CAD build for the part. Positions are in the model's coordinates, mm. Face numbers are marked on the shaded views. A direction names the side the tool comes from. Give positions to 0.01 mm unless a question says otherwise; leave off trailing zeros. Write each loop counter-clockwise with the first axis right and the second up, starting at its lowest first coordinate (ties: lowest second). Pieces come first, ordered by that corner, then holes. Notation, with made-up numbers: (43, 1) - (83, 1) arc R16 ccw to (83, 8) - close; hole circle Ø8 at (46, 48). An arc over 180 degrees is marked (long way). Answer as a JSON object with one key per item and string values.
from build123d import *

# Parameters (mm, degrees)
SKETCH1_W               = 56.4
SKETCH1_H               = 56.4
SKETCH1_R               = 2.5
SKETCH1_R_2             = 20
SKETCH1_W_2             = 42.3
SKETCH1_H_2             = 42.45
SKETCH1_R_3             = 1.25
SKETCH1_R_4             = 12.5
BOSS_EXTRUDE1_DEPTH     = 3
BOSS_EXTRUDE2_DEPTH     = 3
BOSS_EXTRUDE3_DEPTH     = 3
BOSS_EXTRUDE4_DEPTH     = 3
BOSS_EXTRUDE5_DEPTH     = 7.05
SKETCH6_W               = 62.4
SKETCH6_H               = 25
BOSS_EXTRUDE6_DEPTH     = 3
SKETCH7_W               = 55.35
SKETCH7_H               = 25
BOSS_EXTRUDE7_DEPTH     = 3
SKETCH8_W               = 26.348542459
SKETCH8_H               = 5
SKETCH8_W_2             = 28.376425856
SKETCH8_W_3             = 30.843971631
SKETCH8_W_4             = 29.425531915
BOSS_EXTRUDE8_DEPTH     = 60
SKETCH9_R               = 69.252729773
SKETCH9_R_2             = 19.252729773
CUT_EXTRUDE1_DEPTH      = 5
CUT_EXTRUDE2_START      = -51
SKETCH9_2_R             = 69.252729773
SKETCH9_2_R_2           = 19.252729773
CUT_EXTRUDE2_DEPTH      = 5
CUT_EXTRUDE3_DEPTH      = 136.205325339
CUT_EXTRUDE3_DEPTH_BACK = 136.205325339
SKETCH10_R              = 62.5
BOSS_EXTRUDE9_DEPTH     = 31
CUT_EXTRUDE4_DEPTH      = 129.360741662
CUT_EXTRUDE4_DEPTH_BACK = 129.360741662
SKETCH12_R              = 3


with BuildPart() as part:
    # Sketch1 → Boss-Extrude1 (new body)
    # profile 1 of 2: a face of its own
    with BuildSketch(Plane.XY):
        Rectangle(SKETCH1_W, SKETCH1_H)
        with Locations((-23.55, -23.55)):
            Circle(SKETCH1_R, mode=Mode.SUBTRACT)
        with Locations((-23.55, 23.55)):
            Circle(SKETCH1_R, mode=Mode.SUBTRACT)
        with Locations((23.55, 23.55)):
            Circle(SKETCH1_R, mode=Mode.SUBTRACT)
        with Locations((23.55, -23.55)):
            Circle(SKETCH1_R, mode=Mode.SUBTRACT)
        Circle(SKETCH1_R_2, mode=Mode.SUBTRACT)
    # profile 2 of 2: a face of its own
    with BuildSketch(Plane.XY):
        with Locations((0, 49.425)):
            Rectangle(SKETCH1_W_2, SKETCH1_H_2)
        with Locations((-15.49, 34)):
            Circle(SKETCH1_R_3, mode=Mode.SUBTRACT)
        with Locations((-15.49, 64.99)):
            Circle(SKETCH1_R_3, mode=Mode.SUBTRACT)
        with Locations((15.5, 64.99)):
            Circle(SKETCH1_R_3, mode=Mode.SUBTRACT)
        with Locations((15.5, 34)):
            Circle(SKETCH1_R_3, mode=Mode.SUBTRACT)
        with Locations((0, 49.5)):
            Circle(SKETCH1_R_4, mode=Mode.SUBTRACT)
    extrude(amount=BOSS_EXTRUDE1_DEPTH)

    # Sketch2 → Boss-Extrude2 (add)
    with BuildSketch(Plane.ZY.offset(28.2)):
        Polygon((-22, -28.2), (-30, 28.2), (0, 28.2), (3, 28.2), (3, -28.2), align=None)
    boss_extrude2 = extrude(amount=BOSS_EXTRUDE2_DEPTH)

    # Mirror1: Boss-Extrude2 across plane
    add(boss_extrude2.mirror(Plane(origin=(0, 0, 0), x_dir=(0, 0, 1), z_dir=(1, 0, 0))))

    # Sketch3 → Boss-Extrude3 (add)
    with BuildSketch(Plane(origin=(0, 28.2, 0), x_dir=(1, 0, 0), z_dir=(0, 1, 0))):
        Polygon((-21.1, 30), (-31.2, 30), (-31.2, -3), (31.2, -3), (31.2, 30), (21.1, 30), (21.1, 0), (-21.1, 0), align=None)
    extrude(amount=BOSS_EXTRUDE3_DEPTH)

    # Sketch4 → Boss-Extrude4 (add)
    with BuildSketch(Plane(origin=(21.15, 0, 0), x_dir=(0, 0, -1), z_dir=(1, 0, 0))):
        Polygon((30, 31.2), (22, 70.65), (-3, 70.65), (-3, 31.2), align=None)
    boss_extrude4 = extrude(amount=BOSS_EXTRUDE4_DEPTH)

    # Mirror2: Boss-Extrude4 across plane
    add(boss_extrude4.mirror(Plane(origin=(0, 0, 0), x_dir=(0, 0, 1), z_dir=(1, 0, 0))))

    # Sketch5 → Boss-Extrude5 (add)
    with BuildSketch(Plane(origin=(24.15, 0, 0), x_dir=(0, 0, -1), z_dir=(1, 0, 0))):
        Polygon((-3, 31.2), (30, 31.2), (22, 70.65), (-3, 70.65), align=None)
    extrude(amount=BOSS_EXTRUDE5_DEPTH)

    # Sketch6 → Boss-Extrude6 (add)
    with BuildSketch(Plane.XZ.offset(28.2)):
        with Locations((0, -9.5)):
            Rectangle(SKETCH6_W, SKETCH6_H)
    extrude(amount=BOSS_EXTRUDE6_DEPTH)

    # Sketch7 → Boss-Extrude7 (add)
    with BuildSketch(Plane(origin=(0, 70.65, 0), x_dir=(1, 0, 0), z_dir=(0, 1, 0))):
        with Locations((3.525, 9.5)):
            Rectangle(SKETCH7_W, SKETCH7_H)
    extrude(amount=BOSS_EXTRUDE7_DEPTH)

    # Sketch8 → Boss-Extrude8 (add)
    with BuildSketch(Plane(origin=(31.2, 0, 0), x_dir=(0, 0, -1), z_dir=(1, 0, 0))):
        with Locations((10.17427123, 61.5)):
            Rectangle(SKETCH8_W, SKETCH8_H)
        with Locations((11.188212928, 51.5)):
            Rectangle(SKETCH8_W_2, SKETCH8_H)
        with Locations((12.421985816, 15.5)):
            Rectangle(SKETCH8_W_3, SKETCH8_H)
        with Locations((11.712765958, 5.5)):
            Rectangle(SKETCH8_W_4, SKETCH8_H)
    extrude(amount=BOSS_EXTRUDE8_DEPTH)

    # Sketch9 → Cut-Extrude1 (cut)
    with BuildSketch(Plane(origin=(0, 54, 0), x_dir=(1, 0, 0), z_dir=(0, 1, 0))):
        with Locations((70.970898887, -60.264609649)):
            Circle(SKETCH9_R)
        with Locations((70.970898887, -60.264609649)):
            Circle(SKETCH9_R_2, mode=Mode.SUBTRACT)
    extrude(amount=-CUT_EXTRUDE1_DEPTH, mode=Mode.SUBTRACT)

    # Sketch9<2> → Cut-Extrude2 (cut)
    with BuildSketch(Plane(origin=(0, 54, 0), x_dir=(1, 0, 0), z_dir=(0, 1, 0)).offset(CUT_EXTRUDE2_START)):
        with Locations((70.970898887, -60.264609649)):
            Circle(SKETCH9_2_R)
        with Locations((70.970898887, -60.264609649)):
            Circle(SKETCH9_2_R_2, mode=Mode.SUBTRACT)
    extrude(amount=CUT_EXTRUDE2_DEPTH, mode=Mode.SUBTRACT)

    # Sketch10 → Cut-Extrude3 (cut, two sides: drawn at the far end of the back side and taken through both)
    with BuildSketch(Plane(origin=(0, 64, 0), x_dir=(1, 0, 0), z_dir=(0, 1, 0)).offset(-CUT_EXTRUDE3_DEPTH_BACK)):
        with Locations((70.970898887, -60.264609649)):
            Circle(SKETCH10_R)
    extrude(amount=CUT_EXTRUDE3_DEPTH + CUT_EXTRUDE3_DEPTH_BACK, mode=Mode.SUBTRACT)

    # Sketch11 → Boss-Extrude9 (add)
    with BuildSketch(Plane.XZ.offset(-49)):
        with BuildLine():
            Line((46.2, -25.376425856), (76.2, -25.376425856))
            Line((76.2, -25.376425856), (76.2, -8.790419729))
            ThreePointArc((76.2, -8.790419729), (60.957142835, -8.260314799), (46.2, -4.406428299))
            Line((46.2, -4.406428299), (46.2, -25.376425856))
        make_face()
    extrude(amount=BOSS_EXTRUDE9_DEPTH)

    # Sketch12 → Cut-Extrude4 (cut, two sides: drawn at the far end of the back side and taken through both)
    with BuildSketch(Plane(origin=(0, 54, 0), x_dir=(1, 0, 0), z_dir=(0, 1, 0)).offset(-CUT_EXTRUDE4_DEPTH_BACK)):
        with Locations(Location((83.7, 18.348542459, 0), (0, 0, 180))):
            Circle(SKETCH12_R)
        with Locations(Location((38.7, 18.348542459, 0), (0, 0, 180))):
            Circle(SKETCH12_R)
    extrude(amount=CUT_EXTRUDE4_DEPTH + CUT_EXTRUDE4_DEPTH_BACK, mode=Mode.SUBTRACT)


solid = part.part
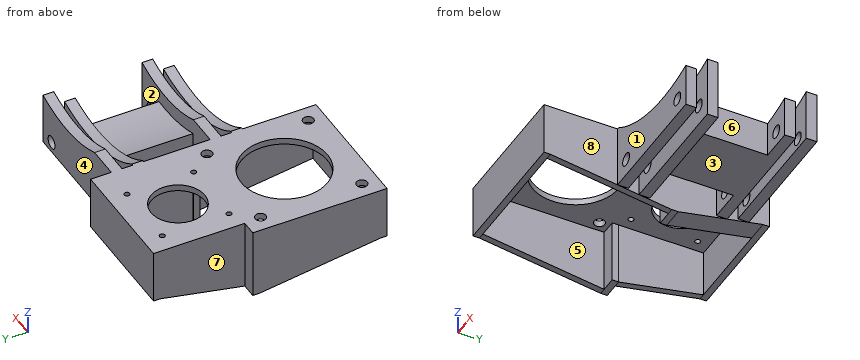
Item 1: Cut at A-A (x = 0). Give the cut face in (y, z), and give its area (3 significant figures).
Entries:
{"outline": "(-31.2, -22) - (-28.2, -22) - (-28.2, 0) - (-20, 0) - (-20, 3) - (-31.2, 3) - close; (20, 0) - (37, 0) - (37, 3) - (20, 3) - close; (62, 0) - (70.65, 0) - (70.65, -22) - (73.65, -22) - (73.65, 3) - (62, 3) - close", "area": "252 mm2"}
Item 2: Mould opens along Y. For the marked faces 1, 2 and 3 say: +Y half, -Y half, draft (parallel to the pull), parting line (faces both ways), or undercut.
Entries:
{"face 1": "-Y half", "face 2": "undercut", "face 3": "draft"}
Item 3: Cut at B-B (y = 0). Give the cut face in (x, z), and give its area (3 significant figures).
Entries:
{"outline": "(-31.2, -26) - (-28.2, -26) - (-28.2, 0) - (-20, 0) - (-20, 3) - (-31.2, 3) - close; (20, 0) - (28.2, 0) - (28.2, -26) - (31.2, -26) - (31.2, 3) - (20, 3) - close", "area": "223 mm2"}
Item 4: Cut at C-C (y = 47.5). Give the cut face in (x, z), and give its area (3 significant figures).
Entries:
{"outline": "(-24.15, -26.69) - (-21.15, -26.69) - (-21.15, 0) - (-12.34, 0) - (-12.34, 3) - (-24.15, 3) - close; (12.34, 0) - (21.15, 0) - (21.15, -26.69) - (31.2, -26.69) - (31.2, 3) - (12.34, 3) - close; (46.2, -25.38) - (76.2, -25.38) - (76.2, -8.79) arc R69.25 cw to (46.2, -4.41) - close", "area": "970 mm2"}
Item 5: Flat gauge pins, fed straight in: P1, Ø8, axis at x = 83.7, z = -18.35, coming from the +Y side; P2, Ø8, axis at x = 60, y = 11, coming from the -Z side; P3, Ø6, axis at x = 53.5, y = 54, coming from the -Z side. Where does each tip first touch, or does it go through?
Entries:
{"P1": "y = 64", "P2": "z = -27.84", "P3": "z = -25.38"}
Item 6: Probe line 1 (X direction, y = 25, z = -22); line 2 (X direction, y = 64.99, z = 1.75); line 3 (Y direction, x = 0, z = 1.5). List the from-to ranges inside material, lowest first. Write a range as from..to.
Entries:
{"line 1": "-31.2..-28.2, 28.2..31.2, 46.2..76.2", "line 2": "-24.15..-16.74, -14.24..14.25, 16.75..31.2", "line 3": "-31.2..-20, 20..37, 62..73.65"}
Item 7: Which spindle directions (+Z, -Z, +X, -X, +Y, -Y) get a long thin tool onto all of the face, cutting with end or side? Do the marked faces 4, 5, 6, 7 and 8. Say none if no direction does.
Entries:
{"face 4": "+Z, -Z, +X, +Y", "face 5": "-Z", "face 6": "+Z, -Z, +X", "face 7": "+Z, -Z, -X, +Y", "face 8": "+Z, -Z, +X, -Y"}
Item 8: Cut at D-D (z = -13.5). State how many separate pieces and enclosed holes the cut face has, and give its area (3 significant figures).
Entries:
{"separate pieces": "1", "enclosed holes": "2", "area": "3,400 mm2"}
